Work out the finished part from the listing and answer in its coordinate system (mm). Face numbers are marked on the shaded views. A direction names the side the tool comes from. Round coordinates to 2 decimals unless told otherwise and drop trailing zeros. Order: outer loops, then holes, each group sorted by start corner. A loop starts at its lowest first (then second) coordinate and runs counter-clockwise, first axis right, second up. Notation, with made-up numbers: (-4, -1.5) - (48, -1.5) arc R20 ccw to (48, 13.5) - close; hole circle Ø7 at (-37, -10.75). An arc over 180 degrees is marked (long way). Use one line per item in the form item = value. Start each with the question number.
Q1. The part is cut by section C-C on y = 8.75. Determine the outline of the cut face in (x, z), plus the area to 3 significant figures.
Q2. Which of the six approach directions +Z, -Z, +X, -X, +Y, -Y give full straight-line access (tool end or side, diameter ignored) to the marked faces 1, 2 and 3?
Q3. The part is cut by section A-A on x = 9.75. Determine the outline of the cut face in (y, z).
Q4. Find the intervals of material crossed by line 1 (X direction, y = 12.7, z = 2.8); line 2 (Z direction, x = 0, y = 8.25); line 3 (Y direction, x = -8.25, z = 8), in increasing order. Write a range as [from, to].
Q5. The part is cut by section B-B on x = 0. Determine the outline of the cut face in (y, z).
Q6. For a pull along X with two mould halves and no side action, classify the marked faces 4, 5 and 6 as +X half, -X half, draft (parallel to the pull), parting line (faces both ways), or undercut.
Q7. The part is cut by section D-D on z = 19.75. Determine the outline of the cut face in (x, y).
Q8. Given P1, Ø10, axis at x = 0, z = 12.7, coming from the +Y side; P2, Ø3, axis at x = -1.5, z = 8, coming from the +Y side; P3, Ø11.5, axis at x = 0, y = 12.7, coming from the +Z side, each flat-ended and moving along its own axis, determine where each tip first touches the part or whether it passes through.
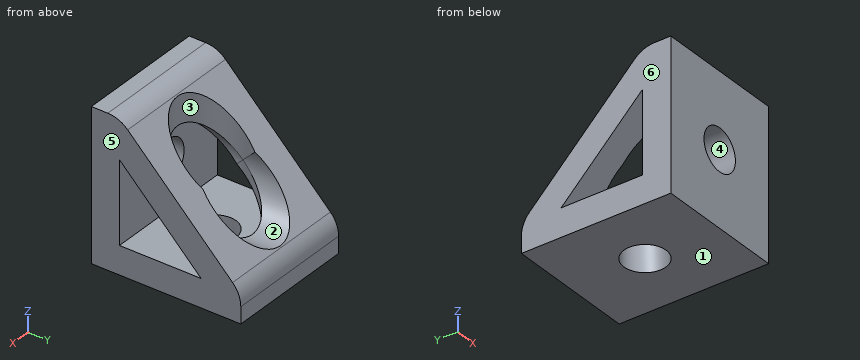
Autodesk Inventor part; units mm, degrees
ref_plane "YZ Plane" through (0, 0, 0) normal (1, 0, 0) x (0, 1, 0)
ref_plane "XZ Plane" through (0, 0, 0) normal (0, 1, 0) x (-1, 0, 0)
ref_plane "XY Plane" through (0, 0, 0) normal (0, 0, 1) x (1, 0, 0)
sketch "Sketch_1" plane through (0, 0, 0) normal (1, 0, 0) x (0, 1, 0)
  line L0 (2.7972, 25.4) -> (0, 25.4)
  line L1 (0, 25.4) -> (0, 0)
  line L2 (0, 0) -> (25.4, 0)
  line L3 (25.4, 0) -> (25.4, 2.7972)
  arc A0 (25.4, 2.7972) -> (24.0014, 6.1738) centre (20.6248, 2.7972) ccw
  line L4 (24.0014, 6.1738) -> (6.1738, 24.0014)
  arc A1 (6.1738, 24.0014) -> (2.7972, 25.4) centre (2.7972, 20.6248) ccw
  line L5 (4.7752, 18.6468) -> (4.7752, 4.7752)
  line L6 (4.7752, 4.7752) -> (18.6468, 4.7752)
  line L7 (18.6468, 4.7752) -> (4.7752, 18.6468)
extrude "Extrusion1" add sketch "Sketch_1" along normal mid plane 22.225
sketch "Sketch2" plane through (-11.1125, 0, 25.4) normal (0, -1, 0) x (1, 0, 0)
  point P0 (11.1125, -12.7)
hole "Hole1" at (0, 0, 12.7) direction (0, 1, 0) diameter 7.1374 depth 4.7752
sketch "Sketch3" plane through (11.1125, 0, 0) normal (0, 0, -1) x (-1, 0, 0)
  point P0 (11.1125, 12.7)
hole "Hole2" at (0, 12.7, 0) direction (0, 0, 1) diameter 7.1374 depth 4.7752
sketch "Sketch_4" plane through (0, 0, 25.4) normal (0, 0, 1) x (1, 0, 0)
  circle A0 centre (0, 12.7) radius 6.35
extrude "Extrusion2" cut sketch "Sketch_4" against normal blind 20.6248
sketch "Sketch_5" plane through (0, 25.4, 0) normal (0, 1, 0) x (1, 0, 0)
  circle A0 centre (0, -12.7) radius 6.35
extrude "Extrusion3" cut sketch "Sketch_5" against normal blind 20.6248
properties part number "4132"
Found:
q1.outline = (-11.11, 0) - (11.11, 0) - (11.11, 4.78) - (-11.11, 4.78) - close; (-11.11, 14.67) - (-6.04, 14.67) arc R6.35 cw to (-4.97, 16.65) - (-4.97, 21.43) - (-11.11, 21.43) - close; (4.97, 16.65) arc R6.35 cw to (6.04, 14.67) - (11.11, 14.67) - (11.11, 21.43) - (4.97, 21.43) - close
q1.area = 187 mm²
q2.face_1 = -Z, +X, -X, +Y, -Y
q2.face_2 = +Y
q2.face_3 = +Z
q3.outline = (0, 0) - (25.4, 0) - (25.4, 2.8) arc R4.78 ccw to (24, 6.17) - (6.17, 24) arc R4.78 ccw to (2.8, 25.4) - (0, 25.4) - close; hole (4.78, 4.78) - (18.65, 4.78) - (4.78, 18.65) - close
q4.line_1 = [-11.11, -3.57], [3.57, 11.11]
q4.line_2 = [0, 4.78]
q4.line_3 = [0, 4.78], [15.42, 22.18]
q5.outline = (0, 0) - (9.13, 0) - (9.13, 4.78) - (4.78, 4.78) - (4.78, 9.13) - (0, 9.13) - close; (0, 16.27) - (4.78, 16.27) - (4.78, 19.05) - (6.35, 19.05) - (6.35, 23.83) - (6.17, 24) arc R4.78 ccw to (2.8, 25.4) - (0, 25.4) - close; (16.27, 0) - (25.4, 0) - (25.4, 2.8) arc R4.78 ccw to (24, 6.17) - (23.83, 6.35) - (19.05, 6.35) - (19.05, 4.78) - (16.27, 4.78) - close
q6.face_4 = undercut
q6.face_5 = +X half
q6.face_6 = -X half
q7.outline = (-11.11, 0) - (11.11, 0) - (11.11, 10.43) - (5.93, 10.43) arc R6.35 cw to (-5.93, 10.43) - (-11.11, 10.43) - close
q8.P1 = 4.78
q8.P2 = 23.68
q8.P3 = 4.78
